Could you check a few things on this model? Use its own coordinates, in mm. A direction names the side the tool comes from. Give positions to 0.01 mm unless a question says otherwise; leave off trailing zeros. Loops run counter-clockwise (first coordinate to the right, second up) from the corner with the lowest first, then second, coordinate; pieces in that order, holes last. Notation, with made-up numbers: (49, 51.25) - (77, 51.25) arc R16 cw to (77, 82.25) - close; hole circle Ø8 at (-19, 5.25). An arc over 180 degrees is marked (long way). Write each question's results on one line, items separated by ' | '. Start each with the question number.
(1) For pin 1 (6.5 mm diameter, centred on y = 7, z = 34, fed in from +X); pin 2 (4 mm diameter, centred on x = 36, y = 4, fed in from +Z), each with a flat end and sliding along its axis, tell me the tip position at first contact or that it passes through.
(2) Suppose I cut it at A-A (z = 25). Please give me the cut outline in (x, y) (3 decimals).
(3) I need wall thicknesses on line 1 (X direction, y = 7.25, z = 14); line 2 (X direction, y = 10.25, z = 31); line 3 (Z direction, x = 51, y = 11.25). Which ranges of each line are inside material? Lowest first, please.
(4) Suppose I cut it at B-B (y = 5.5). Please give me the cut outline in (x, z), and give its area (3 significant figures).
(5) On a 3-axis mill with a long thin cutter (end or side, diameter ignored), from which of +Z, -Z, +X, -X, +Y, -Y can I reach the whole of each face in a straight line? I mean faces 4 (the face through (68.3, 7.9, 25)), 5 (the face through (53.53, 6.26, 13.98)). Say none if no direction works.
(6) If we mould it in two halves opening along X, with no side actions, what happens to faces 1 (the face through (13, 5, 50.8)), 2 (the face through (3.175, 2, 25)), 3 (the face through (19.05, 6, 37))? For each: released by +X, released by -X, zero draft, split by the parting line, or undercut.
(7) Suppose I cut it at C-C (x = 8.5). Please give me the cut outline in (y, z).
(8) Suppose I cut it at D-D (z = 18.5). Please give me the cut outline in (x, y) (3 decimals), and give its area (3 significant figures).
from build123d import *

# Parameters (mm, degrees)
BOSS_EXTRUDE1_DEPTH = 50.8
SKETCH2_W           = 38.1
SKETCH2_H           = 40.64
CUT_EXTRUDE1_DEPTH  = 76.2
FILLET1_R           = 12.7
SKETCH3_OUTSIDE_W   = 96.692
SKETCH3_OUTSIDE_H   = 33.192
SKETCH3_OUTSIDE_W_2 = 69.85
SKETCH3_OUTSIDE_H_2 = 12.7
CUT_EXTRUDE2_DEPTH  = 93.457395594


with BuildPart() as part:
    # Sketch1 → Boss-Extrude1 (new body)
    with BuildSketch(Plane.XY):
        Polygon((0, 0), (76.2, 0), (63.5, 12.7), (12.7, 12.7), align=None)
    extrude(amount=BOSS_EXTRUDE1_DEPTH)

    # Sketch2 → Cut-Extrude1 (cut)
    with BuildSketch(Plane(origin=(0, 12.7, 0), x_dir=(1, 0, 0), z_dir=(0, 1, 0))):
        with Locations((38.1, -30.48)):
            Rectangle(SKETCH2_W, SKETCH2_H)
    extrude(amount=-CUT_EXTRUDE1_DEPTH, mode=Mode.SUBTRACT)

    # Fillet1
    fillet1_edges = [part.edges().sort_by_distance(p)[0] for p in [
        (19.05, 6.35, 10.16),
        (57.15, 6.35, 10.16),
    ]]
    fillet(fillet1_edges, radius=FILLET1_R)

    # Sketch3 outside → Cut-Extrude2 (cut, through all)
    with BuildSketch(Plane(origin=(0, 0, 0), x_dir=(-1, 0, 0), z_dir=(0, 0, -1))):
        with Locations((-38.1, 6.35)):
            Rectangle(SKETCH3_OUTSIDE_W, SKETCH3_OUTSIDE_H)
        with Locations((-38.1, 6.35)):
            Rectangle(SKETCH3_OUTSIDE_W_2, SKETCH3_OUTSIDE_H_2, mode=Mode.SUBTRACT)
    extrude(amount=-CUT_EXTRUDE2_DEPTH, mode=Mode.SUBTRACT)


solid = part.part
Output values:
1) pin 1: x = 72.45 | pin 2: z = 10.16
2) outline: (3.175, 0) - (19.05, 0) - (19.05, 12.7) - (12.7, 12.7) - (3.175, 3.175) - close; (57.15, 0) - (73.025, 0) - (73.025, 3.175) - (63.5, 12.7) - (57.15, 12.7) - close
3) line 1: 7.25 to 22.65, 53.55 to 68.95 | line 2: 10.25 to 19.05, 57.15 to 65.95 | line 3: 0 to 11.98
4) outline: (5.5, 0) - (70.7, 0) - (70.7, 50.8) - (57.15, 50.8) - (57.15, 22.86) arc R12.7 cw to (44.45, 10.16) - (31.75, 10.16) arc R12.7 cw to (19.05, 22.86) - (19.05, 50.8) - (5.5, 50.8) - close | area: 1,830 mm2
5) face 4: +Z, -Z, +X, +Y | face 5: +Z, +Y, -Y
6) face 1: zero draft | face 2: released by -X | face 3: undercut
7) outline: (0, 0) - (8.5, 0) - (8.5, 50.8) - (0, 50.8) - close
8) outline: (3.175, 0) - (19.822, 0) - (19.822, 12.7) - (12.7, 12.7) - (3.175, 3.175) - close; (56.378, 0) - (73.025, 0) - (73.025, 3.175) - (63.5, 12.7) - (56.378, 12.7) - close | area: 332 mm2
